Geometry: final body of the model. Coordinates: model frame, mm. A direction names the side the tool comes from. Give positions to 0.01 mm unless a question says otherwise; leave off trailing zeros. Loops run counter-clockwise (first coordinate to the right, second up) from the corner with the lowest first, then second, coordinate; pieces in that order, holes last.
from build123d import *

# Parameters (mm, degrees)
SKETCH1_R           = 5
BOSS_EXTRUDE1_DEPTH = 10
SKETCH2_R           = 5
BOSS_EXTRUDE2_DEPTH = 15
SKETCH3_W           = 5
SKETCH3_H           = 260
BOSS_EXTRUDE3_DEPTH = 45
SKETCH8_W           = 5
SKETCH8_H           = 19
BOSS_EXTRUDE4_DEPTH = 20
SKETCH9_W           = 19
SKETCH9_H           = 10
SKETCH9_H_2         = 20
BOSS_EXTRUDE5_DEPTH = 45
SKETCH10_W          = 19
SKETCH10_H          = 40
BOSS_EXTRUDE6_DEPTH = 10
BOSS_EXTRUDE7_DEPTH = 5


with BuildPart() as part:
    # Sketch1 → Boss-Extrude1 (new body)
    with BuildSketch(Plane.XY):
        with BuildLine():
            Line((-5, -20), (5, -20))
            ThreePointArc((5, -20), (19.142135624, -14.142135624), (25, 0))
            Line((25, 0), (25, 260))
            ThreePointArc((25, 260), (19.142135624, 274.142135624), (5, 280))
            Line((5, 280), (-5, 280))
            ThreePointArc((-5, 280), (-19.142135624, 274.142135624), (-25, 260))
            Line((-25, 260), (-25, 0))
            ThreePointArc((-25, 0), (-19.142135624, -14.142135624), (-5, -20))
        make_face()
        Circle(SKETCH1_R, mode=Mode.SUBTRACT)
    boss_extrude1 = extrude(amount=BOSS_EXTRUDE1_DEPTH)

    # Sketch2 → Boss-Extrude2 (add)
    with BuildSketch(Plane.XY.offset(10)):
        with Locations((0, 260)):
            Circle(SKETCH2_R)
    boss_extrude2 = extrude(amount=BOSS_EXTRUDE2_DEPTH)

    # Sketch3 → Boss-Extrude3 (add)
    with BuildSketch(Plane(origin=(0, 0, 0), x_dir=(-1, 0, 0), z_dir=(0, 0, -1))):
        with Locations((22.5, 130)):
            Rectangle(SKETCH3_W, SKETCH3_H)
    boss_extrude3 = extrude(amount=BOSS_EXTRUDE3_DEPTH)

    # Mirror1: Boss-Extrude1, Boss-Extrude2, Boss-Extrude3 across plane
    add(boss_extrude1.mirror(Plane.XY.offset(-45)))
    add(boss_extrude2.mirror(Plane.XY.offset(-45)))
    add(boss_extrude3.mirror(Plane.XY.offset(-45)))

    # Sketch8 → Boss-Extrude4 (add)
    with BuildSketch(Plane.XZ):
        with Locations((-22.5, -39.5)):
            Rectangle(SKETCH8_W, SKETCH8_H)
    extrude(amount=BOSS_EXTRUDE4_DEPTH)

    # Sketch9 → Boss-Extrude5 (add)
    with BuildSketch(Plane(origin=(-20, 0, 0), x_dir=(0, 0, -1), z_dir=(1, 0, 0))):
        with Locations((39.5, -15)):
            Rectangle(SKETCH9_W, SKETCH9_H)
        with Locations((39.5, 40)):
            Rectangle(SKETCH9_W, SKETCH9_H_2)
    extrude(amount=BOSS_EXTRUDE5_DEPTH)

    # Sketch10 → Boss-Extrude6 (add)
    with BuildSketch(Plane(origin=(-20, 0, 0), x_dir=(0, 0, -1), z_dir=(1, 0, 0))):
        with Locations((39.5, 10)):
            Rectangle(SKETCH10_W, SKETCH10_H)
    extrude(amount=BOSS_EXTRUDE6_DEPTH)

    # Sketch11 → Boss-Extrude7 (add)
    with BuildSketch(Plane.ZY.offset(25)):
        Polygon((10, 0), (-30, 0), (-30, -20), (-49, -20), (-49, 0), (-100, 0), (-100, 260), (10, 260), align=None)
    extrude(amount=BOSS_EXTRUDE7_DEPTH)


solid = part.part
Item 1: Ray query, probe 1 along Z at (x, y) = (22, 122); probe 2 along Y at (x, z) = (0, -93.25); probe 3 along Z at (x, y) = (-17.5, -3). Return the intervals inside material, ascending.
Values follow:
probe 1: z = -100 to -90, 0 to 10
probe 2: y = -20 to -5, 5 to 280
probe 3: z = -100 to -90, -49 to -30, 0 to 10
Item 2: Section query C-C on y = 174.5. Return loops of the section in (x, z), plus the area to 3 significant figures.
Values follow:
outline: (-30, -100) - (25, -100) - (25, -90) - (-20, -90) - (-20, 0) - (25, 0) - (25, 10) - (-30, 10) - close
area: 2,000 mm2
Item 3: Section query D-D on x = 13. Return loops of the section in (y, z).
Values follow:
outline: (-20, -49) - (-10, -49) - (-10, -30) - (-20, -30) - close; (-18.33, -100) - (278.33, -100) - (278.33, -90) - (-18.33, -90) - close; (-18.33, 0) - (278.33, 0) - (278.33, 10) - (-18.33, 10) - close; (30, -49) - (50, -49) - (50, -30) - (30, -30) - close
Item 4: Set-up query: faces 5 (the face through (-14, 15, -30)), 6 (the face through (18.986, -14.297, 4.93)), 7 (the face through (-19.297, -13.986, 4.93)), 8 (the face through (-19.297, -13.986, -94.93)). Return all of +Z, -Z, +X, -X, +Y, -Y with unobstructed straight access to the full face (end or side cutting, diameter ignored); none if empty.
Values follow:
face 5: +X, -Y
face 6: +Z, +X, -Y
face 7: +Z, -X, -Y
face 8: -Z, -X, -Y
Item 5: Pin query (flat end, axial travel): pin 1 (5 mm diameter, centred on x = -27, z = -35.5, fed in from +Y); pin 2 (1.5 mm diameter, centred on x = -22, y = 21, fed in from -Z); pin 3 (21 mm diameter, centred on y = 6.5, z = -38.5, fed in from +X). Return the tip coordinate at first contact, or that it passes through.
Values follow:
pin 1: stops at y = 260
pin 2: stops at z = -100
pin 3: stops at x = -10
Item 6: Draft query along Y for faces 1 (the face through (2, 50, -39)), 2 (the face through (-10, 10, -39)), 3 (the face through (-1.08, -4.88, -94.93)), 4 (the face through (-25, 0, -74)). Return one class per face: +Y half, -Y half, draft (parallel to the pull), parting line (faces both ways), or undercut.
Values follow:
face 1: +Y half
face 2: undercut
face 3: undercut
face 4: -Y half
Item 7: Section query B-B on z = -41. Return loops of the section in (x, y), plus the area to 3 significant figures.
Values follow:
outline: (-30, -20) - (25, -20) - (25, -10) - (-10, -10) - (-10, 30) - (25, 30) - (25, 50) - (-20, 50) - (-20, 260) - (-30, 260) - close
area: 4,550 mm2
Item 8: Section query A-A on x = 0. Give the number of separate pieces and of enclosed holes in the cut face, plus the area to 3 significant figures.
Values follow:
separate pieces: 6
enclosed holes: 0
area: 6,670 mm2
